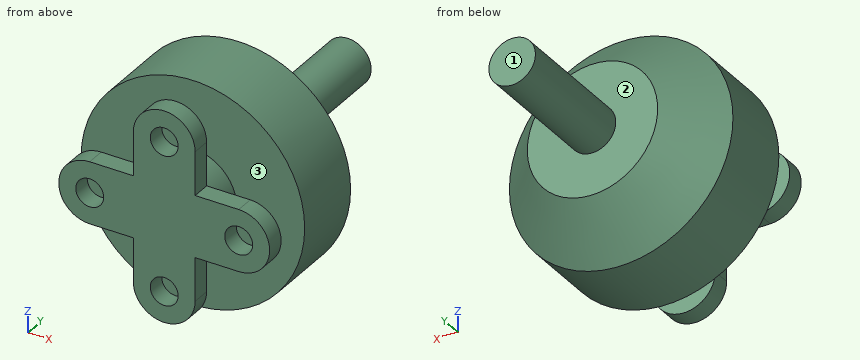
from build123d import *

# Parameters (mm, degrees)
SKETCH_1_R      = 1.5
EXTRUDE_1_DEPTH = 2
SKETCH_2_R      = 4.695496225
EXTRUDE_2_DEPTH = 3
SKETCH_3_R      = 12
EXTRUDE_3_DEPTH = 13
CHAMFER_1_SIZE  = 5
SKETCH_4_R      = 2.5
EXTRUDE_4_DEPTH = 14


with BuildPart() as part:
    # 草图1 → 凸台-拉伸1 (new body)
    with BuildSketch(Plane(origin=(0, 0, 0), x_dir=(1, 0, 0), z_dir=(0, 1, 0))):
        with BuildLine():
            Line((-3.320217222, -4.320217222), (-3.320217222, -8))
            ThreePointArc((-3.320217222, -8), (0, -11.320217222), (3.320217222, -8))
            Line((3.320217222, -8), (3.320217222, -4.320217222))
            Line((3.320217222, -4.320217222), (3.320217222, -3.320217222))
            Line((3.320217222, -3.320217222), (4.320217222, -3.320217222))
            Line((4.320217222, -3.320217222), (8, -3.320217222))
            ThreePointArc((8, -3.320217222), (11.320217222, 0), (8, 3.320217222))
            Line((8, 3.320217222), (4.320217222, 3.320217222))
            Line((4.320217222, 3.320217222), (3.320217222, 3.320217222))
            Line((3.320217222, 3.320217222), (3.320217222, 4.320217222))
            Line((3.320217222, 4.320217222), (3.320217222, 8))
            ThreePointArc((3.320217222, 8), (0, 11.320217222), (-3.320217222, 8))
            Line((-3.320217222, 8), (-3.320217222, 4.320217222))
            Line((-3.320217222, 4.320217222), (-3.320217222, 3.320217222))
            Line((-3.320217222, 3.320217222), (-4.320217222, 3.320217222))
            Line((-4.320217222, 3.320217222), (-8, 3.320217222))
            ThreePointArc((-8, 3.320217222), (-11.320217222, 0), (-8, -3.320217222))
            Line((-8, -3.320217222), (-4.320217222, -3.320217222))
            Line((-4.320217222, -3.320217222), (-3.320217222, -3.320217222))
            Line((-3.320217222, -3.320217222), (-3.320217222, -4.320217222))
        make_face()
        with Locations((0, -8)):
            Circle(SKETCH_1_R, mode=Mode.SUBTRACT)
        with Locations((8, 0)):
            Circle(SKETCH_1_R, mode=Mode.SUBTRACT)
        with Locations((-8, 0)):
            Circle(SKETCH_1_R, mode=Mode.SUBTRACT)
        with Locations((0, 8)):
            Circle(SKETCH_1_R, mode=Mode.SUBTRACT)
    extrude(amount=EXTRUDE_1_DEPTH)

    # 草图2 → 凸台-拉伸2 (add)
    with BuildSketch(Plane(origin=(0, 2, 0), x_dir=(1, 0, 0), z_dir=(0, 1, 0))):
        Circle(SKETCH_2_R)
    extrude(amount=EXTRUDE_2_DEPTH)

    # 草图3 → 凸台-拉伸3 (add)
    with BuildSketch(Plane(origin=(0, 5, 0), x_dir=(1, 0, 0), z_dir=(0, 1, 0))):
        Circle(SKETCH_3_R)
    extrude(amount=EXTRUDE_3_DEPTH)

    # 倒角1
    chamfer_1_edges = [part.edges().sort_by_distance(p)[0] for p in [
        (-12, 18, 0),
    ]]
    chamfer(chamfer_1_edges, length=CHAMFER_1_SIZE)

    # 草图4 → 凸台-拉伸4 (add)
    with BuildSketch(Plane(origin=(0, 18, 0), x_dir=(1, 0, 0), z_dir=(0, 1, 0))):
        Circle(SKETCH_4_R)
    extrude(amount=EXTRUDE_4_DEPTH)


solid = part.part
Design review of the part built by this model. Coordinates are the model's own, in mm. Face numbers are marked on the shaded views. A direction names the side the tool comes from. Coordinates: 2 decimals unless noted, no trailing zeros. Order: outer loops, then holes, each group sorted by start corner. A loop starts at its lowest first (then second) coordinate and runs counter-clockwise, first axis right, second up.
Item 1: For pin 1 Ø1 at (y, z) = (1.5, -6) entering from -X; pin 2 Ø5 at (y, z) = (5, -8) entering from +X; pin 3 Ø5.5 at (x, z) = (-6.5, 1) entering from +Y; pin 4 Ø10 at (y, z) = (22.5, 9.5) entering from -X, all flat-tipped, find the tip position at first contact; note any pin that passes through.
Item 2: For the marked faces 1, 2 and 3, list the 3-axis set-ups (+Z, -Z, +X, -X, +Y, -Y) from which the entire face can be reached by the end or side of a thin tool; tool diameter is ignored.
Item 3: Take a section at B-B, the plane x = 0.25. Count the separate pieces of the cut face and the enclosed holes in it, then the cut area to 3 significant figures.
Item 4: Take a section at A-A, the plane z = 0. Write out the cut boundary in (x, y).
Item 5: Take a section at C-C, the plane y = 2.5. Write out the cut boundary in (x, z), then the cut area to 3 significant figures.
Item 6: For line 1 (X direction, y = 1, z = 0); line 2 (X direction, y = 0.75, z = -8), list the stretches that pass through material, from the lowest coordinate up.
Item 7: Take a section at D-D, the plane y = 17. Write out the cut boundary in (x, z), then the cut area to 3 significant figures.
The answers:
1. pin 1: stops at x = -3.32
1. pin 2: stops at x = 10.67
1. pin 3: stops at y = 18
1. pin 4: passes through
2. face 1: +Z, -Z, +X, -X, +Y
2. face 2: +Y
2. face 3: none
3. separate pieces: 3
3. enclosed holes: 0
3. area: 418 mm2
4. outline: (-12, 5) - (-4.7, 5) - (-4.7, 2) - (-6.5, 2) - (-6.5, 0) - (6.5, 0) - (6.5, 2) - (4.7, 2) - (4.7, 5) - (12, 5) - (12, 13) - (7, 18) - (2.5, 18) - (2.5, 32) - (-2.5, 32) - (-2.5, 18) - (-7, 18) - (-12, 13) - close; (-11.32, 0) - (-9.5, 0) - (-9.5, 2) - (-11.32, 2) - close; (9.5, 0) - (11.32, 0) - (11.32, 2) - (9.5, 2) - close
5. outline: circle Ø9.39 at (0, 0)
5. area: 69.3 mm2
6. line 1: x = -11.32 to -9.5, -6.5 to 6.5, 9.5 to 11.32
6. line 2: x = -3.32 to -1.5, 1.5 to 3.32
7. outline: circle Ø16 at (0, 0)
7. area: 201 mm2
